Input: part model. Units: mm. Frame: model coordinates. Face numbers are marked on the shaded views. Round coordinates to 2 decimals unless told otherwise and drop trailing zeros. Order: outer loops, then holes, each group sorted by start corner. A loop starts at its lowest first (then second) coordinate and runs counter-clockwise, first axis right, second up. Notation, with made-up numbers: (80.5, 59.25) - (138.5, 59.25) arc R16 ccw to (138.5, 80.25) - close; hole circle Ø3 at (11.25, 79.5). An arc over 180 degrees is marked (long way). One line per item, written item: value. Start each with the question number.
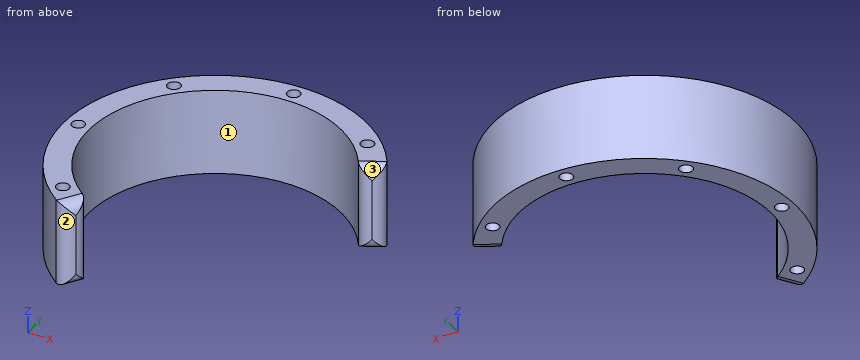
from build123d import *

# Parameters (mm, degrees)
SKETCH_2_R          = 60
SKETCH_2_R_2        = 2.6
SKETCH_2_R_3        = 50
EXTRUDE_1_DEPTH     = 34
CUT_EXTRUDE_START   = -34
SKETCH_3_R          = 2.6
CUT_EXTRUDE_1_DEPTH = 34
FILLET_1_R          = 5


with BuildPart() as part:
    # 草图2 → 凸台-拉伸1 (new body)
    with BuildSketch(Plane.XY):
        Circle(SKETCH_2_R)
        with Locations((0, 55)):
            Circle(SKETCH_2_R_2, mode=Mode.SUBTRACT)
        with Locations((38.890872965, 38.890872965)):
            Circle(SKETCH_2_R_2, mode=Mode.SUBTRACT)
        with Locations((55, 0)):
            Circle(SKETCH_2_R_2, mode=Mode.SUBTRACT)
        with Locations((38.890872965, -38.890872965)):
            Circle(SKETCH_2_R_2, mode=Mode.SUBTRACT)
        with Locations((0, -55)):
            Circle(SKETCH_2_R_2, mode=Mode.SUBTRACT)
        with Locations((-38.890872965, -38.890872965)):
            Circle(SKETCH_2_R_2, mode=Mode.SUBTRACT)
        with Locations((-55, 0)):
            Circle(SKETCH_2_R_2, mode=Mode.SUBTRACT)
        with Locations((-38.890872965, 38.890872965)):
            Circle(SKETCH_2_R_2, mode=Mode.SUBTRACT)
        Circle(SKETCH_2_R_3, mode=Mode.SUBTRACT)
    extrude(amount=EXTRUDE_1_DEPTH)

    # 草图3 → 切除-拉伸1 (cut)
    with BuildSketch(Plane.XY.offset(34).offset(CUT_EXTRUDE_START)):
        with BuildLine():
            Line((53.220649991, 27.704916794), (44.350541659, 23.087430662))
            ThreePointArc((44.350541659, 23.087430662), (48.567103491, 11.884294616), (50, 0))
            ThreePointArc((50, 0), (24.049438446, -43.836337785), (-26.864980417, -42.169572291))
            Line((-26.864980417, -42.169572291), (-32.237976501, -50.603486749))
            ThreePointArc((-32.237976501, -50.603486749), (28.859326135, -52.603605342), (60, 0))
            ThreePointArc((60, 0), (58.280524189, 14.26115354), (53.220649991, 27.704916794))
        make_face()
        with Locations((0, -55)):
            Circle(SKETCH_3_R, mode=Mode.SUBTRACT)
        with Locations((38.890872965, -38.890872965)):
            Circle(SKETCH_3_R, mode=Mode.SUBTRACT)
        with Locations((55, 0)):
            Circle(SKETCH_3_R, mode=Mode.SUBTRACT)
    extrude(amount=CUT_EXTRUDE_1_DEPTH, mode=Mode.SUBTRACT)

    # 圆角1
    fillet_1_edges = [part.edges().sort_by_distance(p)[0] for p in [
        (-26.864980417, -42.169572291, 17),
        (48.785595825, 25.396173728, 34),
        (44.350541659, 23.087430662, 17),
        (53.220649991, 27.704916794, 17),
        (-29.551478459, -46.38652952, 0),
        (-32.237976501, -50.603486749, 17),
        (48.785595825, 25.396173728, 0),
        (-29.551478459, -46.38652952, 34),
    ]]
    fillet(fillet_1_edges, radius=FILLET_1_R - 0.0001)  # a hair under: the kernel refuses the full size


solid = part.part
Item 1: Line query: L1, parallel to Y at x = 0, z = 19.5; L2, parallel to Y at x = -32.5, z = 7; L3, parallel to Y at x = -24.5, z = 7.5. Output: solid intervals per line, ascending.
Item 2: Section query D-D on z = 2.5. Return loops of the section in (x, y).
Item 3: Section query B-B on x = 0. Return loops of the section in (y, z), and give its area (3 significant figures).
Item 4: First-contact query: pin 1 Ø5 at (x, z) = (25.5, 10.5) entering from -Y; pin 2 Ø4.5 at (x, y) = (38.89, 38.89) entering from +Z; pin 3 Ø6 at (x, z) = (29, 11) entering from -Y; pin 4 Ø12 at (y, z) = (3.5, 17.5) entering from -X. Flat tips, straight axial feed; report the tip coordinate or a pass-through.
Item 5: Section query C-C on z = 22.5. Give the number of separate pieces and of enclosed holes in the cut face, and give its area (3 significant figures).
Item 6: Pull-direction query (X, two-part tool) for the marked faces 1, 2 and 3; classes: released by +X, released by -X, zero draft, split by the parting line, or undercut.
Item 7: Section query A-A on y = 0. Return loops of the section in (x, z), and give its area (3 significant figures).
Geometry results:
1. L1: y = 50 to 52.4, 57.6 to 60
1. L2: y = -48.37 to -38, 38 to 50.44
1. L3: y = 43.59 to 54.77
2. outline: (-36.7, -47.46) arc R5 ccw to (-31.34, -47.94) - (-28.65, -43.73) arc R5 ccw to (-30.59, -39.55) arc R50 cw (long way) to (42.07, 27.02) arc R5 ccw to (46.06, 24.73) - (50.49, 27.04) arc R5 ccw to (50.48, 32.43) arc R60 ccw (long way) to start; hole circle Ø5.2 at (-55, 0); hole circle Ø5.2 at (-38.89, -38.89); hole circle Ø5.2 at (-38.89, 38.89); hole circle Ø5.2 at (0, 55); hole circle Ø5.2 at (38.89, 38.89)
3. outline: (50, 0) - (52.4, 0) - (52.4, 34) - (50, 34) - close; (57.6, 0) - (60, 0) - (60, 34) - (57.6, 34) - close
3. area: 163 mm^2
4. pin 1: stops at y = 41.42
4. pin 2: passes through
4. pin 3: stops at y = 38.42
4. pin 4: stops at x = -60
5. separate pieces: 1
5. enclosed holes: 5
5. area: 1,890 mm^2
6. face 1: undercut
6. face 2: split by the parting line
6. face 3: released by +X
7. outline: (-60, 0) - (-57.6, 0) - (-57.6, 34) - (-60, 34) - close; (-52.4, 0) - (-50, 0) - (-50, 34) - (-52.4, 34) - close
7. area: 163 mm^2
